```python
from build123d import *

# Parameters (mm, degrees)
BOSS_EXTRUDE1_DEPTH = 40.64
SKETCH2_R           = 3.175
CUT_EXTRUDE1_DEPTH  = 40.64
SKETCH3_W           = 76.2
SKETCH3_H           = 15.24
CUT_EXTRUDE2_DEPTH  = 40.64


with BuildPart() as part:
    # Sketch1 → Boss-Extrude1 (new body)
    with BuildSketch(Plane(origin=(0, 0, 0), x_dir=(1, 0, 0), z_dir=(0, 1, 0))):
        with BuildLine():
            Line((31.75, 101.6), (31.75, 107.95))
            ThreePointArc((31.75, 107.95), (9.299359697, 98.650640303), (0, 76.2))
            Line((0, 76.2), (0, 0))
            Line((0, 0), (6.35, 0))
            Line((6.35, 0), (6.35, 76.2))
            ThreePointArc((6.35, 76.2), (13.789487758, 94.160512242), (31.75, 101.6))
        make_face()
    extrude(amount=BOSS_EXTRUDE1_DEPTH)

    # Sketch2 → Cut-Extrude1 (cut)
    with BuildSketch(Plane(origin=(6.35, 0, 0), x_dir=(0, 0, -1), z_dir=(1, 0, 0))):
        with Locations((6.35, 7.62)):
            Circle(SKETCH2_R)
    extrude(amount=-CUT_EXTRUDE1_DEPTH, mode=Mode.SUBTRACT)

    # Sketch3 → Cut-Extrude2 (cut)
    with BuildSketch(Plane(origin=(0, 0, 0), x_dir=(0, 0, -1), z_dir=(1, 0, 0))):
        with Locations((50.8, 7.62)):
            Rectangle(SKETCH3_W, SKETCH3_H)
    extrude(amount=CUT_EXTRUDE2_DEPTH, mode=Mode.SUBTRACT)


solid = part.part
```
CAD build for the part. Positions are in the model's coordinates, mm. A direction names the side the tool comes from. Coordinates: 2 decimals unless noted, no trailing zeros. Write each loop counter-clockwise with the first axis right and the second up, starting at its lowest first coordinate (ties: lowest second). Pieces come first, ordered by that corner, then holes.
(1) Cut at B-B, the plane y = 7.62. List the corners of the cut face in (x, z) (3 decimals).
(2) Cut at C-C, the plane y = 29. List the corners of the cut face in (x, z).
(3) Drill centre lines: probe 1 along Z at (x, y) = (4, 5); probe 2 along Y at (x, z) = (2, -6); probe 3 along X at (y, z) = (31, -70). Where is each one in solid material? Low to high.
(4) Two-plate mould, pull along Z, no slides. Class faces 1 (the face through (9.55, 20.04, -98.9)), 2 (the face through (4, 15.24, -50)), 3 (the face through (3.22, 5.69, -3.83)), 4 (the face through (0, 25, -39)): +Z half, -Z half, draft (parallel to the pull), parting line (faces both ways), or undercut.
(5) Flat gauge pins, fed straight in: pin 1 (2 mm diameter, centred on x = 27.5, y = 30, fed in from -Z); pin 2 (7.5 mm diameter, centred on y = 7.62, z = -6.35, fed in from +X); pin 3 (3 mm diameter, centred on x = 3.5, z = -52.5, fed in from -Y); pin 4 (12 mm diameter, centred on x = 22.5, z = -90, fed in from +Y). Where does each tip first touch, or does it go through?
(6) Cut at A-A, the plane z = -6.35. List the corners of the cut face in (x, y) (3 decimals), and give its area (3 significant figures).
(7) 3-axis set-ups, long thin cutter, end or side, ignore diameter. For faces 5 (the face through (6.35, 25, -38)), 6 (the face through (6, 8, -88.9)), 7 (the face through (17, 0, -98)): which of +Z, -Z, +X, -X, +Y, -Y reach the whole face in a straight line?
(8) Cut at D-D, the plane x = 23. List the corners of the cut face in (y, z).
Geometry says:
1. outline: (0, -12.7) - (6.35, -12.7) - (6.35, -9.525) - (0, -9.525) - close; (0, -3.175) - (6.35, -3.175) - (6.35, 0) - (0, 0) - close; (2.651, -88.9) arc R31.75 ccw to (31.75, -107.95) - (31.75, -101.6) arc R25.4 cw to (9.753, -88.9) - close
2. outline: (0, -76.2) arc R31.75 ccw to (31.75, -107.95) - (31.75, -101.6) arc R25.4 cw to (6.35, -76.2) - (6.35, 0) - (0, 0) - close
3. probe 1: z = -91.63 to -88.9, -12.7 to -8.14, -4.56 to 0
3. probe 2: y = 0 to 4.46, 10.78 to 40.64
3. probe 3: x = 0 to 6.35
4. face 1: -Z half
4. face 2: undercut
4. face 3: undercut
4. face 4: draft
5. pin 1: stops at z = -107.78
5. pin 2: stops at x = 6.35
5. pin 3: stops at y = 15.24
5. pin 4: passes through
6. outline: (0, 0) - (6.35, 0) - (6.35, 4.445) - (0, 4.445) - close; (0, 10.795) - (6.35, 10.795) - (6.35, 40.64) - (0, 40.64) - close
6. area: 218 mm2
7. face 5: +Z, +X, +Y, -Y
7. face 6: +X, -X, -Y
7. face 7: +Z, -Z, +X, -X, -Y
8. outline: (0, -106.72) - (40.64, -106.72) - (40.64, -100.05) - (0, -100.05) - close
